Input: part model. Units: mm. Frame: model coordinates. Round coordinates to 2 decimals unless told otherwise and drop trailing zeros. Loops run counter-clockwise (first coordinate to the right, second up) from the corner with the lowest first, then second, coordinate; pieces in that order, holes last.
1) First-contact query: pin 1 (4 mm diameter, centred on x = 5, y = 5, fed in from +Z); pin 2 (2.5 mm diameter, centred on x = 5, y = -5, fed in from -Z). Flat tips, straight axial feed; report the tip coordinate or a pass-through.
2) Draft query along Y for faces 1 (the face through (0, 0, 2)), 2 (the face through (0, -8, 1)), 3 (the face through (5.806, 3.735, 0.986)), 4 (the face through (-6.11, 3.99, 0.99)). Return one class per face: pulls with the +Y half, pulls with the -Y half, needs draft (parallel to the pull), parting line crosses it, or undercut.
3) Section A-A, the plane y = 5. Return loops of the section in (x, z), and give its area (3 significant figures).
4) Ray query, line 1 along X through (y, z) = (-5, 0.6); line 2 along X through (y, z) = (5.75, 1.2). Return the intervals inside material, ascending.
5) Section C-C, the plane z = 0.4. Return loops of the section in (x, y).
Autodesk Fusion 360 part; units mm, degrees
sketch "Skizze1" plane through (0, 0, 0) normal (0, 0, 1) x (1, 0, 0)
  line L0 (5, -5) -> (-5, -5)
  circle A0 centre (-5, -5) radius 1.5
  line L1 (-5, -5) -> (-5, 5)
  circle A1 centre (-5, 5) radius 1.5
  line L2 (5, 5) -> (5, -5)
  line L3 (-5, 5) -> (5, 5)
  circle A2 centre (5, 5) radius 1.5
  circle A3 centre (5, -5) radius 1.5
  line L4 (-8, 8) -> (8, 8)
  line L5 (8, 8) -> (8, -8)
  line L6 (8, -8) -> (-8, -8)
  line L7 (-8, -8) -> (-8, 8)
  dimension "d1" = 10
  dimension "d2" = 10
  dimension "d3" = 3
  dimension "d4" = 3
  dimension "d5" = 3
  dimension "d6" = 3
  dimension "d7" = 16
  dimension "d8" = 16
extrude "Extrusion1" add sketch "Skizze1" along normal blind 2 contours L0 A0 L1 A1 L2 L3 A2 A3 | L4 L5 L6 L7
Final values:
1. pin 1: stops at z = 2
1. pin 2: passes through
2. face 1: needs draft
2. face 2: pulls with the -Y half
2. face 3: undercut
2. face 4: undercut
3. outline: (-8, 0) - (-6.5, 0) - (-6.5, 2) - (-8, 2) - close; (-3.5, 0) - (3.5, 0) - (3.5, 2) - (-3.5, 2) - close; (6.5, 0) - (8, 0) - (8, 2) - (6.5, 2) - close
3. area: 20.0 mm2
4. line 1: x = -8 to -6.5, -3.5 to 3.5, 6.5 to 8
4. line 2: x = -8 to -6.3, -3.7 to 3.7, 6.3 to 8
5. outline: (-8, -8) - (8, -8) - (8, 8) - (-8, 8) - close; hole circle Ø3 at (-5, -5); hole circle Ø3 at (-5, 5); hole circle Ø3 at (5, -5); hole circle Ø3 at (5, 5)
